Input: part model. Units: mm. Frame: model coordinates. A direction names the side the tool comes from. Coordinates: 2 decimals unless noted, no trailing zeros. Write each loop counter-clockwise with the first axis right and the second up, starting at its lowest first coordinate (ties: lowest second). Pieces come first, ordered by that corner, then holes. Notation, with made-up numbers: (72, 39) -> (107, 39) arc R15 ccw to (107, 48) -> close; hole circle Ø6 at (51, 25.25). An arc over 180 degrees is marked (long way). Use one line per item in the form item = value. Start each with the question number.
(1) Cut plane D-D on y = -15. Return the cut outline in (x, z), plus the area to 3 significant figures.
(2) Ray query, line 1 along Y through (x, z) = (-2, 0.8); line 2 along X through (y, z) = (7.5, 0.45); line 3 along Y through (x, z) = (-0.75, 0.35). Return the intervals inside material, ascending.
(3) Cut plane B-B on z = 0.3. Return the cut outline in (x, y).
(4) Pull-direction query (Y, two-part tool) for faces 3 (the face through (0, 18, 1)), 4 (the face through (-10.5, 1, 1)), 5 (the face through (1.75, 2, 1)); classes: released by +Y, released by -Y, zero draft, split by the parting line, or undercut.
(5) Set-up query: faces 1 (the face through (-3, 6.75, 1)), 2 (the face through (-2, 0, 0)). Return all of +Z, -Z, +X, -X, +Y, -Y with unobstructed straight access to the full face (end or side cutting, diameter ignored); none if empty.
(6) Cut plane C-C on y = 0. Return the cut outline in (x, z), plus the area to 3 significant figures.
(7) Cut plane A-A on x = 3. Return the cut outline in (y, z).
```python
from build123d import *

# Parameters (mm, degrees)
F0_W       = 21
F0_H       = 36
F1_DEPTH   = 2
F2_SIZE    = 2
F3_SIZE2   = 8
F3_SIZE    = 5
F3_2_SIZE2 = 8
F3_2_SIZE  = 5
F4_R       = 1.7


with BuildPart() as f1:
    # F0 (on Top) → F1 (new body)
    with BuildSketch(Plane.XY):
        Rectangle(F0_W, F0_H)
        Polygon((1.75, 3.25), (1.75, -0.5), (-1.75, -0.5), (-1.75, 3.25), (-5.5, 3.25), (-5.5, 6.75), (-1.75, 6.75), (-1.75, 10.5), (1.75, 10.5), (1.75, 6.75), (5.5, 6.75), (5.5, 3.25), align=None, mode=Mode.SUBTRACT)
    extrude(amount=F1_DEPTH)

    # F2
    f2_edges = [f1.edges().sort_by_distance(p)[0] for p in [
        (10.5, 18, 1),
        (-10.5, 18, 1),
    ]]
    chamfer(f2_edges, length=F2_SIZE)

    # F3
    f3_edges = [f1.edges().sort_by_distance(p)[0] for p in [
        (10.5, -18, 1),
    ]]
    f3_side = f1.faces().sort_by_distance((10.5, -1, 1))[0]
    chamfer(f3_edges, length=F3_SIZE, length2=F3_SIZE2, reference=f3_side)

    # F3#2
    f3_2_edges = [f1.edges().sort_by_distance(p)[0] for p in [
        (-10.5, -18, 1),
    ]]
    f3_2_side = f1.faces().sort_by_distance((-10.5, -1, 1))[0]
    chamfer(f3_2_edges, length=F3_2_SIZE, length2=F3_2_SIZE2, reference=f3_2_side)

    # F4
    f4_edges = [f1.edges().sort_by_distance(p)[0] for p in [
        (5.5, 6.75, 1),
        (1.75, 10.5, 1),
        (-1.75, 10.5, 1),
        (-5.5, 6.75, 1),
        (-5.5, 3.25, 1),
        (-1.75, -0.5, 1),
        (1.75, -0.5, 1),
        (5.5, 3.25, 1),
    ]]
    fillet(f4_edges, radius=F4_R)


solid = f1.part
```
Values:
q1.outline = (-7.3, 0) -> (7.3, 0) -> (7.3, 2) -> (-7.3, 2) -> close
q1.area = 29.2 mm2
q2.line_1 = -18 to 3.25, 6.75 to 18
q2.line_2 = -10.5 to -1.75, 1.75 to 10.5
q2.line_3 = -18 to -0.35, 10.35 to 18
q3.outline = (-10.5, -13) -> (-2.5, -18) -> (2.5, -18) -> (10.5, -13) -> (10.5, 16) -> (8.5, 18) -> (-8.5, 18) -> (-10.5, 16) -> close; hole (-5.5, 4.95) arc R1.7 ccw to (-3.8, 3.25) -> (-1.75, 3.25) -> (-1.75, 1.2) arc R1.7 ccw to (-0.05, -0.5) -> (0.05, -0.5) arc R1.7 ccw to (1.75, 1.2) -> (1.75, 3.25) -> (3.8, 3.25) arc R1.7 ccw to (5.5, 4.95) -> (5.5, 5.05) arc R1.7 ccw to (3.8, 6.75) -> (1.75, 6.75) -> (1.75, 8.8) arc R1.7 ccw to (0.05, 10.5) -> (-0.05, 10.5) arc R1.7 ccw to (-1.75, 8.8) -> (-1.75, 6.75) -> (-3.8, 6.75) arc R1.7 ccw to (-5.5, 5.05) -> close
q4.face_3 = released by +Y
q4.face_4 = zero draft
q4.face_5 = undercut
q5.face_1 = +Z, -Z
q5.face_2 = -Z, +X, -X, +Y, -Y
q6.outline = (-10.5, 0) -> (-1.25, 0) -> (-1.25, 2) -> (-10.5, 2) -> close; (1.25, 0) -> (10.5, 0) -> (10.5, 2) -> (1.25, 2) -> close
q6.area = 37.0 mm2
q7.outline = (-17.69, 0) -> (3.25, 0) -> (3.25, 2) -> (-17.69, 2) -> close; (6.75, 0) -> (18, 0) -> (18, 2) -> (6.75, 2) -> close
